Source: CAD feature listing. Evaluate the final solid. Frame: model axes, mm. Face numbers are marked on the shaded views. Round coordinates to 2 decimals unless told otherwise and drop trailing zeros.
from build123d import *

# Parameters (mm, degrees)
SWEEP_1_PROFILE_R   = 12
SWEEP_1_PROFILE_R_2 = 10


with BuildPart() as part:
    # 扫描-薄件1: sweep along a curve in space
    with BuildLine() as sweep_1_path:
        Line((-293.907053201, -176.904078828, 0), (-215.210942182, -51.240174508, 0))
        ThreePointArc((-215.210942182, -51.240174508, 0), (-206.832168677, -42.47680964, 0), (-195.669049964, -37.745510677, 0))
        Line((-195.669049964, -37.745510677, 0), (-112.434772166, -21.097592117, 0))
        ThreePointArc((-83.45170927, -16.323468261, -23.798598546), (-93.844250534, -17.667130883, -6.69804309), (-112.434772166, -21.097592117, 0))
        Line((-83.45170927, -16.323468261, -23.798598546), (-67.801697088, -16.323468261, -96.628223589))
        ThreePointArc((-67.801697088, -16.323468261, -96.628223589), (-70.278739917, -16.323468261, -116.306023698), (-84.49226654, -16.323468261, -130.138131969))
        Line((-84.49226654, -16.323468261, -130.138131969), (-258.992373197, -16.323468261, -211.207155939))
    # 扫描-薄件1 profile (on start of the path) → 扫描-薄件1 (sweep)
    with BuildSketch(Plane(origin=(-293.907053201, -176.904078828, 0), x_dir=(0.8475245838768447, -0.5307561396012122, 0), z_dir=(0.5307561396012122, 0.8475245838768447, 0))):
        Circle(SWEEP_1_PROFILE_R)
        Circle(SWEEP_1_PROFILE_R_2, mode=Mode.SUBTRACT)
    sweep(path=sweep_1_path.line)


solid = part.part
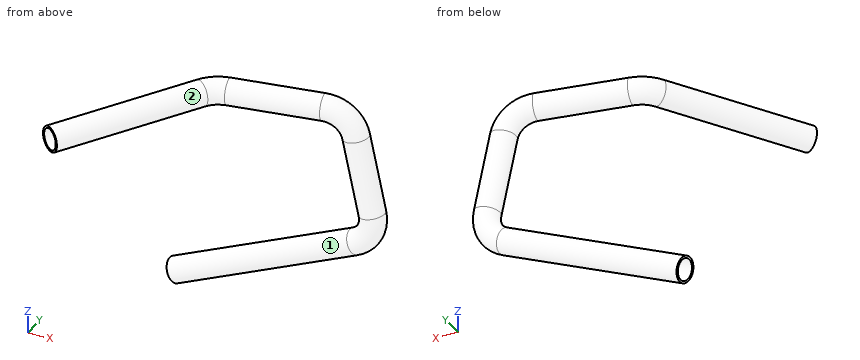
1) Section query A-A on x = -220. State how many separate pieces and enclosed holes the cut face has, then the cut area to 3 significant figures.
Taken from the geometry:
separate pieces: 2
enclosed holes: 2
area: 399 mm2
2) Pull-direction query (Z, two-part tool) for the marked faces 1 and 2; classes: released by +Z, released by -Z, zero draft, split by the parting line, or undercut.
Taken from the geometry:
face 1: undercut
face 2: split by the parting line
3) Material intervals for line 1 (Z direction, x = -146.5, y = -22); line 2 (Y direction, x = -166, z = -166); line 3 (Y direction, x = -136.5, z = -147.5), sorted ascending.
Taken from the geometry:
line 1: z = -170.6 to -168.02, -149.87 to -147.29, -10.51 to -8.15, 8.15 to 10.51
line 2: y = -28.18 to -26.16, -6.49 to -4.46
line 3: y = -26.62 to -24.2, -8.45 to -6.03
4) Contact query for flat-ended pins moving along their axis: P1, Ø5, axis at x = -266.5, y = -145.5, coming from the +Z side; P2, Ø6, axis at x = -249, z = -17, coming from the +Y side (3 decimals); P3, Ø8, axis at x = -102.5, z = -130, coming from the +Y side. Output: stop coordinate, or through.
Taken from the geometry:
P1: stops at z = 11.29
P2: passes through
P3: stops at y = -4.91
